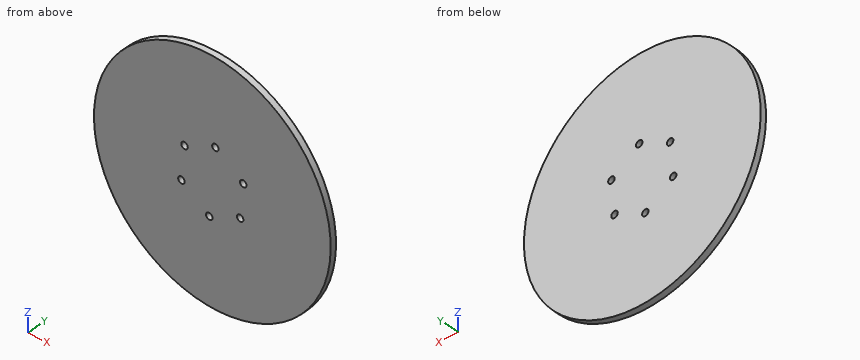
from build123d import *

# Parameters (mm, degrees)
SKETCH_2_R          = 60
EXTRUDE_1_DEPTH     = 3
CUT_EXTRUDE_1_DEPTH = 10


with BuildPart() as part:
    # 草图2 → 凸台-拉伸1 (new body)
    with BuildSketch(Plane(origin=(0, 0, 0), x_dir=(1, 0, 0), z_dir=(0, 1, 0))):
        with Locations(Location((0, 0, 0), (0, 0, 270))):
            Circle(SKETCH_2_R)
    extrude(amount=EXTRUDE_1_DEPTH)

    # 草图3 → 切除-拉伸1 (cut)
    with BuildSketch(Plane.XZ):
        with BuildLine():
            ThreePointArc((17.005273727, 6.290323162), (16.607301875, 8.589587915), (14.308037122, 8.191616063))
            ThreePointArc((14.308037122, 8.191616063), (14.706008974, 5.89235131), (17.005273727, 6.290323162))
        make_face()
        with BuildLine():
            ThreePointArc((15.447809647, -10.88922298), (15.049837795, -8.589958227), (12.750573042, -8.987930079))
            ThreePointArc((12.750573042, -8.987930079), (13.148544894, -11.287194832), (15.447809647, -10.88922298))
        make_face()
        with BuildLine():
            ThreePointArc((-0.208845777, -18.130192593), (-0.606817629, -15.830927839), (-2.906082382, -16.228899691))
            ThreePointArc((-2.906082382, -16.228899691), (-2.50811053, -18.528164444), (-0.208845777, -18.130192593))
        make_face()
        with BuildLine():
            ThreePointArc((-14.308037122, -8.191616063), (-14.706008974, -5.89235131), (-17.005273727, -6.290323162))
            ThreePointArc((-17.005273727, -6.290323162), (-16.607301875, -8.589587915), (-14.308037122, -8.191616063))
        make_face()
        with BuildLine():
            ThreePointArc((-12.750573042, 8.987930079), (-13.148544894, 11.287194832), (-15.447809647, 10.88922298))
            ThreePointArc((-15.447809647, 10.88922298), (-15.049837795, 8.589958227), (-12.750573042, 8.987930079))
        make_face()
        with BuildLine():
            ThreePointArc((2.906082382, 16.228899691), (2.50811053, 18.528164444), (0.208845777, 18.130192593))
            ThreePointArc((0.208845777, 18.130192593), (0.606817629, 15.830927839), (2.906082382, 16.228899691))
        make_face()
    extrude(amount=-CUT_EXTRUDE_1_DEPTH, mode=Mode.SUBTRACT)


solid = part.part
Verification items for the finished model (mm, model axes). Coordinates: 2 decimals unless noted, no trailing zeros. Order: outer loops, then holes, each group sorted by start corner. A loop starts at its lowest first (then second) coordinate and runs counter-clockwise, first axis right, second up. Notation, with made-up numbers: M 74,-20.5 L 106,-20.5 A25 cw 106,-8.5 Z; hole C 54,75 d4. An arc over 180 degrees is marked long. Write each question's results on one line, items separated by ' | '.
1) Section check A-A on y = 1. Record the cut outline in (x, z), plus the area to 3 significant figures.
Solved:
outline: C 0,0 d120; hole C -15.66,-7.24 d3.3; hole C -14.1,9.94 d3.3; hole C -1.56,-17.18 d3.3; hole C 1.56,17.18 d3.3; hole C 14.1,-9.94 d3.3; hole C 15.66,7.24 d3.3 | area: 11,300 mm²
2) Section check C-C on x = 52.5. Record the cut outline in (y, z), plus the area to 3 significant figures.
Solved:
outline: M 0,-29.05 L 3,-29.05 L 3,29.05 L 0,29.05 Z | area: 174 mm²
3) Scan lines: line 1 along Z through (x, y) = (-15, 0.2); line 2 along Z through (x, y) = (-2.5, 1.75); line 3 along X through (y, z) = (0.95, 11). Record each from-to range of solid material in increasing order. Write a range as [from, to].
Solved:
line 1: z = [-58.09, -8.75], [-5.73, 8.56], [11.32, 58.09] | line 2: z = [-59.95, -18.53], [-15.83, 59.95] | line 3: x = [-58.98, -15.36], [-12.84, 58.98]
4) Section check B-B on x = -43. Record the cut outline in (y, z), plus the area to 3 significant figures.
Solved:
outline: M 0,-41.84 L 3,-41.84 L 3,41.84 L 0,41.84 Z | area: 251 mm²
